Geometry: final body of the model. Coordinates: model frame, mm. A direction names the side the tool comes from. Round coordinates to 2 decimals unless told otherwise and drop trailing zeros. Order: outer loops, then holes, each group sorted by start corner. A loop starts at its lowest first (then second) coordinate and runs counter-clockwise, first axis right, second up. Notation, with made-up numbers: M -9,41.5 L 5,41.5 A18 cw 5,55.5 Z; hole C 42,8 d9. An arc over 180 degrees is marked long. Put each result on its own line as item: value. Start each with the question number.
1) Section A-A, the plane z = -4.25. Return loops of the section in (x, y), then the cut area to 3 significant figures.
2) Access query for faces 1 (the flat face through (-81, 10.989, -5)), 2 (the flat face through (-84.142, -1, -5)), 3 (the flat face through (-81, -12.011, -5)), 4 (the flat face through (-80.142, -1, -5)). Directions: +Z, -Z, +X, -X, +Y, -Y. A direction counts if a zero-diameter tool reaches every point of the face in a straight line with its end or side. Return the directions, or none.
3) Section D-D, the plane y = 19. Return loops of the section in (x, z), then the cut area to 3 significant figures.
4) First-contact query: P1, Ø3, axis at x = -54.5, y = -13, coming from the -Z side; P2, Ø6.5, axis at x = -80.5, z = -3.5, coming from the +Y side; P3, Ø0.6, axis at x = -81.5, z = -4, coming from the -Y side. Flat tips, straight axial feed; report the tip coordinate or a pass-through.
5) Section B-B, the plane y = 6.5. Return loops of the section in (x, z).
6) Draft query along Y for faces 5 (the flat face through (-81, 0, 0)), 6 (the flat face through (-89.142, -1, 1)), 7 (the flat face through (-59, 30.489, 1)). Return one class per face: pulls with the +Y half, pulls with the -Y half, needs draft (parallel to the pull), parting line crosses it, or undercut.
7) Material intervals for probe 1 along X at (y, z) = (-2.5, -4.5); probe 2 along Z at (x, y) = (-36, -15), sorted ascending. Write a range as [from, to].
8) Section C-C, the plane x = -59. Return loops of the section in (y, z), then the cut area to 3 significant figures.
from build123d import *

# Parameters (mm, degrees)
CROQUIS1_W              = 62
CROQUIS1_H              = 62
CROQUIS1_R              = 1.5
SALIENTE_EXTRUIR1_DEPTH = 2
CROQUIS2_W              = 6
CROQUIS2_H              = 23
CROQUIS2_W_2            = 2
CROQUIS2_H_2            = 20.5
SALIENTE_EXTRUIR2_DEPTH = 10


with BuildPart() as part:
    # Croquis1 → Saliente-Extruir1 (new body)
    with BuildSketch(Plane.XY):
        with Locations((-58.141884519, -0.511173184)):
            Rectangle(CROQUIS1_W, CROQUIS1_H)
        with Locations((-85.641884519, 26.988826816)):
            Circle(CROQUIS1_R, mode=Mode.SUBTRACT)
        with Locations((-30.641884519, 26.988826816)):
            Circle(CROQUIS1_R, mode=Mode.SUBTRACT)
        with Locations((-30.641884519, -28.011173184)):
            Circle(CROQUIS1_R, mode=Mode.SUBTRACT)
        with Locations((-85.641884519, -28.011173184)):
            Circle(CROQUIS1_R, mode=Mode.SUBTRACT)
    extrude(amount=SALIENTE_EXTRUIR1_DEPTH)

    # Croquis2 → Saliente-Extruir2 (add)
    with BuildSketch(Plane(origin=(0, 0, 0), x_dir=(-1, 0, 0), z_dir=(0, 0, -1))):
        with Locations((81.141884519, -0.511173184)):
            Rectangle(CROQUIS2_W, CROQUIS2_H)
        with Locations((81.141884519, -0.511173184)):
            Rectangle(CROQUIS2_W_2, CROQUIS2_H_2, mode=Mode.SUBTRACT)
    extrude(amount=SALIENTE_EXTRUIR2_DEPTH)


solid = part.part
Result sheet:
1. outline: M -84.14,-12.01 L -78.14,-12.01 L -78.14,10.99 L -84.14,10.99 Z; hole M -82.14,-10.76 L -80.14,-10.76 L -80.14,9.74 L -82.14,9.74 Z
1. area: 97.0 mm2
2. face 1: -Z, +X, -X, +Y
2. face 2: -Z, -X, +Y, -Y
2. face 3: -Z, +X, -X, -Y
2. face 4: -Z
3. outline: M -89.14,0 L -27.14,0 L -27.14,2 L -89.14,2 Z
3. area: 124 mm2
4. P1: stops at z = 0
4. P2: stops at y = 10.99
4. P3: stops at y = -12.01
5. outline: M -89.14,0 L -84.14,0 L -84.14,-10 L -82.14,-10 L -82.14,0 L -80.14,0 L -80.14,-10 L -78.14,-10 L -78.14,0 L -27.14,0 L -27.14,2 L -89.14,2 Z
6. face 5: undercut
6. face 6: needs draft
6. face 7: pulls with the +Y half
7. probe 1: x = [-84.14, -82.14], [-80.14, -78.14]
7. probe 2: z = [0, 2]
8. outline: M -31.51,0 L 30.49,0 L 30.49,2 L -31.51,2 Z
8. area: 124 mm2
